```python
from build123d import *

# Parameters (mm, degrees)
SKETCH1_W           = 42
SKETCH1_H           = 42
SKETCH1_R           = 1.25
BOSS_EXTRUDE1_DEPTH = 6
CUT_EXTRUDE1_DEPTH  = 31.298514815
BOSS_EXTRUDE2_START = 4.75
SKETCH3_R           = 3.5
SKETCH3_R_2         = 1.25
BOSS_EXTRUDE2_DEPTH = 4.75
SKETCH4_R           = 1.5
CUT_EXTRUDE2_DEPTH  = 31.298514815
CUT_EXTRUDE3_DEPTH  = 2.3


with BuildPart() as part:
    # Sketch1 → Boss-Extrude1 (new body)
    with BuildSketch(Plane.XY):
        Rectangle(SKETCH1_W, SKETCH1_H)
        with Locations((-14, 14)):
            Circle(SKETCH1_R, mode=Mode.SUBTRACT)
        with Locations((14, 14)):
            Circle(SKETCH1_R, mode=Mode.SUBTRACT)
        with Locations((14, -14)):
            Circle(SKETCH1_R, mode=Mode.SUBTRACT)
        with Locations((-14, -14)):
            Circle(SKETCH1_R, mode=Mode.SUBTRACT)
    extrude(amount=-BOSS_EXTRUDE1_DEPTH)

    # Sketch2 → Cut-Extrude1 (cut, through all)
    with BuildSketch(Plane.XY):
        with BuildLine():
            Line((-3.631627179, -10.198790609), (3.631230455, -10.198790609))
            ThreePointArc((3.631230455, -10.198790609), (6.681814195, -13.249374349), (3.631230455, -16.29995809))
            Line((3.631230455, -16.29995809), (-3.631627179, -16.29995809))
            ThreePointArc((-3.631627179, -16.29995809), (-6.68221092, -13.249374349), (-3.631627179, -10.198790609))
        make_face()
    extrude(amount=-CUT_EXTRUDE1_DEPTH, mode=Mode.SUBTRACT)

    # Sketch3 → Boss-Extrude2 (add)
    # profile 1 of 4: a face of its own
    with BuildSketch(Plane.XY.offset(BOSS_EXTRUDE2_START)):
        with Locations(Location((-14, 14, 0), (0, 0, 180))):
            Circle(SKETCH3_R)
        with Locations((-14, 14)):
            Circle(SKETCH3_R_2, mode=Mode.SUBTRACT)
    # profile 2 of 4: a face of its own
    with BuildSketch(Plane.XY.offset(BOSS_EXTRUDE2_START)):
        with Locations(Location((14, 14, 0), (0, 0, 180))):
            Circle(SKETCH3_R)
        with Locations((14, 14)):
            Circle(SKETCH3_R_2, mode=Mode.SUBTRACT)
    # profile 3 of 4: a face of its own
    with BuildSketch(Plane.XY.offset(BOSS_EXTRUDE2_START)):
        with Locations(Location((-14, -14, 0), (0, 0, 180))):
            Circle(SKETCH3_R)
        with Locations((-14, -14)):
            Circle(SKETCH3_R_2, mode=Mode.SUBTRACT)
    # profile 4 of 4: a face of its own
    with BuildSketch(Plane.XY.offset(BOSS_EXTRUDE2_START)):
        with Locations(Location((14, -14, 0), (0, 0, 180))):
            Circle(SKETCH3_R)
        with Locations((14, -14)):
            Circle(SKETCH3_R_2, mode=Mode.SUBTRACT)
    extrude(amount=-BOSS_EXTRUDE2_DEPTH)

    # Sketch4 → Cut-Extrude2 (cut, symmetric)
    with BuildSketch(Plane.XY):
        with Locations((-17.5, -5.882662859)):
            Circle(SKETCH4_R)
        with Locations((-10, 9.117337141)):
            Circle(SKETCH4_R)
        Polygon((-21.661099187, -7.93704977), (-16.848148957, -12.75), (-21.661099187, -17.56295023), align=None)
        Polygon((-21.705309187, 11.072359515), (-11.305917145, 21.471751558), (-21.705309187, 21.471751558), align=None)
    cut_extrude2 = extrude(amount=CUT_EXTRUDE2_DEPTH, both=True, mode=Mode.SUBTRACT)

    # Mirror1: Cut-Extrude2 across plane
    add(cut_extrude2.mirror(Plane(origin=(0, 0, 0), x_dir=(0, 0, 1), z_dir=(1, 0, 0))), mode=Mode.SUBTRACT)

    # Sketch5 → Cut-Extrude3 (cut)
    with BuildSketch(Plane(origin=(0, 0, -6), x_dir=(-1, 0, 0), z_dir=(0, 0, -1))):
        Polygon((-13.222967924, 11.100076814), (-11.100076814, 13.222967924), (-11.87710889, 16.12289111), (-14.777032076, 16.899923186), (-16.899923186, 14.777032076), (-16.12289111, 11.87710889), align=None)
        Polygon((13.222967924, 11.100076814), (16.12289111, 11.87710889), (16.899923186, 14.777032076), (14.777032076, 16.899923186), (11.87710889, 16.12289111), (11.100076814, 13.222967924), align=None)
        Polygon((15.5011107, -16.6), (17.0022214, -14), (15.5011107, -11.4), (12.4988893, -11.4), (10.9977786, -14), (12.4988893, -16.6), align=None)
        Polygon((-15.5011107, -16.6), (-12.4988893, -16.6), (-10.9977786, -14), (-12.4988893, -11.4), (-15.5011107, -11.4), (-17.0022214, -14), align=None)
    extrude(amount=-CUT_EXTRUDE3_DEPTH, mode=Mode.SUBTRACT)


solid = part.part
```
Read the model definition and answer for the solid it produces. Units are mm, in the model's axes. A direction names the side the tool comes from. Coordinates: 2 decimals unless noted, no trailing zeros. Loops run counter-clockwise (first coordinate to the right, second up) from the corner with the lowest first, then second, coordinate; pieces in that order, holes last.
(1) The part is cut by section C-C (y = 8.5). Determine the outline of the cut face in (x, z), and give its area (3 significant figures).
Solution:
outline: (-21, -6) - (-11.37, -6) - (-11.37, 0) - (-21, 0) - close; (-8.63, -6) - (8.63, -6) - (8.63, 0) - (-8.63, 0) - close; (11.37, -6) - (21, -6) - (21, 0) - (11.37, 0) - close
area: 219 mm2
(2) Flat-ended cylindrical pins translate along their axes: pin 1 Ø3.5 at (x, y) = (17.5, -5.88) entering from +Z; pin 2 Ø2.5 at (x, z) = (-14, -5.5) entering from +Y; pin 3 Ø3 at (x, y) = (14, 14) entering from -Z. Find the tip coordinate at first contact, or state that the pin passes through.
Solution:
pin 1: stops at z = 0
pin 2: stops at y = 20.03
pin 3: stops at z = -3.7
(3) The part is cut by section D-D (x = 14). Determine the outline of the cut face in (y, z).
Solution:
outline: (-21, -6) - (-16.6, -6) - (-16.6, -3.7) - (-15.25, -3.7) - (-15.25, 4.75) - (-17.5, 4.75) - (-17.5, 0) - (-21, 0) - close; (-12.75, -3.7) - (-11.4, -3.7) - (-11.4, -6) - (11.31, -6) - (11.31, -3.7) - (12.75, -3.7) - (12.75, 4.75) - (10.5, 4.75) - (10.5, 0) - (-10.5, 0) - (-10.5, 4.75) - (-12.75, 4.75) - close; (15.25, -3.7) - (16.69, -3.7) - (16.69, -6) - (18.78, -6) - (18.78, 0) - (17.5, 0) - (17.5, 4.75) - (15.25, 4.75) - close
(4) The part is cut by section B-B (z = 1). Determine the outline of the cut face in (x, y), and give its area (3 significant figures).
Solution:
outline: (-17.44, -13.34) arc R3.5 ccw (long way) to (-17.14, -12.46) - (-16.85, -12.75) - close; (-17.04, 15.74) arc R3.5 ccw (long way) to (-15.74, 17.04) - close; (15.74, 17.04) arc R3.5 ccw (long way) to (17.04, 15.74) - close; (16.85, -12.75) - (17.14, -12.46) arc R3.5 ccw (long way) to (17.44, -13.34) - close; hole circle Ø2.5 at (-14, -14); hole circle Ø2.5 at (-14, 14); hole circle Ø2.5 at (14, -14); hole circle Ø2.5 at (14, 14)
area: 134 mm2
(5) The part is cut by section A-A (x = 3). Determine the outline of the cut face in (y, z), and give its area (3 significant figures).
Solution:
outline: (-21, -6) - (-16.3, -6) - (-16.3, 0) - (-21, 0) - close; (-10.2, -6) - (21, -6) - (21, 0) - (-10.2, 0) - close
area: 215 mm2
(6) The mould has two halves that part along Y. Classify faces 1 (the face through (21, -19, -3)), 2 (the face through (-13.347, 16.517, -4.866)), 3 (the face through (0, 21, -3)): released by +Y, released by -Y, zero draft, split by the parting line, or undercut.
Solution:
face 1: zero draft
face 2: undercut
face 3: released by +Y
(7) Consider line 1 along Y through (x, z) = (14, 2.75); line 2 along X through (y, z) = (14.5, 2.25); line 3 along Y through (x, z) = (-10, -2.8). Determine where each line is inside the solid, lowest interval first.
Solution:
line 1: y = -17.5 to -15.25, -12.75 to -10.5, 10.5 to 12.75, 15.25 to 17.5
line 2: x = -17.46 to -15.15, -12.85 to -10.54, 10.54 to 12.85, 15.15 to 17.46
line 3: y = -21 to 7.62, 10.62 to 21
(8) A tool of negligible diameter and unlimited length cuts with its end or side. For faces 4 (the face through (19, -10.6, -3.1)), 5 (the face through (15.824, 15.853, -4.866)), 6 (the face through (-19, -10.6, -3.1)), from which of +Z, -Z, +X, -X, +Y, -Y can it reach the whole face along a straight path? Write none if from no direction.
Solution:
face 4: +Z, -Z, +X
face 5: -Z
face 6: +Z, -Z, -X
